Geometry: final body of the model. Coordinates: model frame, mm. Round coordinates to 2 decimals unless told otherwise and drop trailing zeros. Loops run counter-clockwise (first coordinate to the right, second up) from the corner with the lowest first, then second, coordinate; pieces in that order, holes last. Notation, with made-up numbers: M 50.5,47 L 99.5,47 A18 ccw 99.5,65 Z; hole C 11,22.25 d9. An arc over 180 degrees is marked long. Return JSON: item names as keys, results as strings.
from build123d import *

# Parameters (mm, degrees)
F2_R = 3
F3_R = 2


with BuildPart() as f1:
    # F0 (on Front) → F1 (revolve)
    with BuildSketch(Plane.XZ):
        Polygon((-50.205132, 15), (-50.205132, 0), (299.794868, 0), (299.794868, 5.5), (99.794868, 5.5), (99.794868, 15), align=None)
    revolve(axis=Axis((124.794868, 0, 0), (-1, 0, 0)))

    # F2
    f2_edges = [f1.edges().sort_by_distance(p)[0] for p in [
        (299.794868, 0, -5.5),
    ]]
    fillet(f2_edges, radius=F2_R)

    # F3
    f3_edges = [f1.edges().sort_by_distance(p)[0] for p in [
        (99.794868, 0, -15),
        (-50.205132, 0, -15),
    ]]
    fillet(f3_edges, radius=F3_R)


solid = f1.part
Q1. Section query B-B (x = 38). Output: boundary loops of the cut face in (y, z), plus the area to 3 significant figures.
Determined:
{"outline": "C 0,0 d30", "area": "707 mm^2"}
Q2. Pull-direction query (Y, two-part tool) for faces 1 (the flat face through (99.795, 0, -6)), 2 (the cylindrical face through (196.92, -5.37, -1.19)); classes: pulls with the +Y half, pulls with the -Y half, needs draft (parallel to the pull), parting line crosses it, or undercut.
Determined:
{"face 1": "needs draft", "face 2": "parting line crosses it"}
Q3. Pin query (flat end, axial travel): pin 1 (3 mm diameter, centred on x = 142, z = -5, fed in from +Y); pin 2 (10 mm diameter, centred on x = 53, y = -10.5, fed in from +Z); pin 3 (4 mm diameter, centred on x = 77, z = -9, fed in from +Y). Return the tip coordinate at first contact, or that it passes through.
Determined:
{"pin 1": "stops at y = 4.24", "pin 2": "stops at z = 13.96", "pin 3": "stops at y = 13.27"}
Q4. Section query A-A (x = 127). Output: boundary loops of the cut face in (y, z).
Determined:
{"outline": "C 0,0 d11"}
Q5. Material intervals for L1, parallel to X at y = -10, z = -3.25; L2, parallel to X at y = -0.5, z = -3; L3, parallel to Z at x = 89.5, y = 0.5, sorted ascending.
Determined:
{"L1": "x = -50.21 to 99.79", "L2": "x = -50.21 to 299.75", "L3": "z = -14.99 to 14.99"}
